Verification items for the finished model (mm, model axes). Round coordinates to 2 decimals unless told otherwise and drop trailing zeros. Write each loop counter-clockwise with the first axis right and the second up, starting at its lowest first coordinate (ties: lowest second). Pieces come first, ordered by that corner, then holes. Notation, with made-up numbers: (46.25, 53) - (51.25, 53) arc R24 cw to (51.25, 69) - close; hole circle Ø6 at (-12, 82.5). An arc over 180 degrees is marked (long way). Answer as a JSON object with one key per item and string values. Group by question number.
1) Go/stop test with flat-tipped pins: pin 1 Ø1.2 at (x, z) = (57, 2.5) entering from +Y; pin 2 Ø1.5 at (x, z) = (29, 0.5) entering from -Y; pin 3 Ø1.5 at (y, z) = (52, 1.5) entering from -X. Record where each tip stops, or that it passes through.
2) Section check C-C (y = 71). Enter the section's corners in (x, z), then the cut area to 3 significant figures.
3) Section check B-B (x = 34.5). Enter the section's corners in (y, z).
4) Thickness scan on line 1 (X direction, y = 21, z = 0.9); line 2 (Y direction, x = 51, z = 3.45); line 3 (X direction, y = 17.5, z = 1.1). Record the ranges inside material, lowest first.
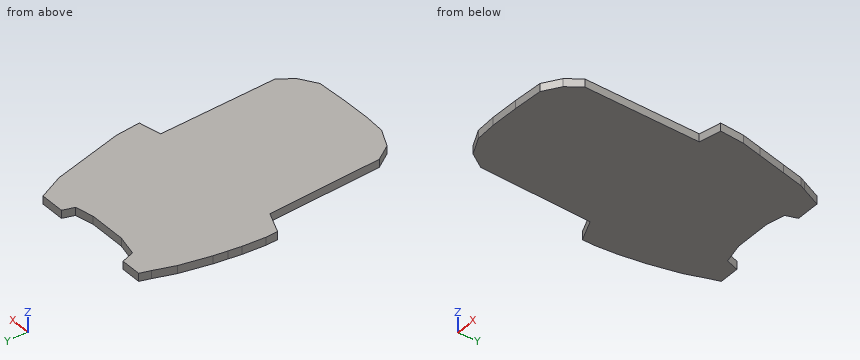
Autodesk Inventor part; units mm, degrees
ref_plane "YZ Plane" through (0, 0, 0) normal (1, 0, 0) x (0, 1, 0)
ref_plane "XZ Plane" through (0, 0, 0) normal (0, 1, 0) x (-1, 0, 0)
ref_plane "XY Plane" through (0, 0, 0) normal (0, 0, 1) x (1, 0, 0)
sketch "Sketch1" plane through (0, 0, 0) normal (0, 0, 1) x (1, 0, 0)
  line L0 (26.9534, 140.31) -> (36.8306, 140.31)
  line L1 (36.8306, 140.31) -> (38.8061, 134.065)
  line L2 (38.8061, 134.065) -> (49.002, 131.6435)
  line L3 (49.002, 131.6435) -> (58.0509, 131.6435)
  line L4 (58.0509, 131.6435) -> (66.8448, 131.6435)
  line L5 (66.8448, 131.6435) -> (75.6388, 133.5552)
  line L6 (75.6388, 133.5552) -> (77.526, 139.065)
  line L7 (77.526, 139.065) -> (89.2513, 139.065)
  line L8 (89.2513, 139.065) -> (93.4636, 129.481)
  line L9 (93.4636, 129.481) -> (94.6369, 126.8115)
  line L10 (94.6369, 126.8115) -> (96.9293, 116.2664)
  line L11 (96.9293, 116.2664) -> (99.976, 102.2517)
  line L12 (99.976, 102.2517) -> (102.1542, 92.2318)
  line L13 (102.1542, 92.2318) -> (102.8007, 80.352)
  line L14 (102.8007, 80.352) -> (92.1232, 78.0307)
  line L15 (92.1232, 78.0307) -> (92.1232, 20.902)
  line L16 (92.1232, 20.902) -> (86.9727, 14.0196)
  line L17 (86.9727, 14.0196) -> (78.9304, 8.8886)
  line L18 (78.9304, 8.8886) -> (64.5453, 8.1057)
  line L19 (64.5453, 8.1057) -> (50.4611, 7.8467)
  line L20 (50.4611, 7.8467) -> (40.2944, 8.4971)
  line L21 (40.2944, 8.4971) -> (31.1734, 13.0172)
  line L22 (31.1734, 13.0172) -> (26.2605, 20.7176)
  line L23 (26.2605, 20.7176) -> (25.2413, 76.1313)
  line L24 (25.2413, 76.1313) -> (14.3454, 80.8506)
  line L25 (14.3454, 80.8506) -> (14.3454, 86.7328)
  line L26 (14.3454, 86.7328) -> (15.5218, 97.7359)
  line L27 (15.5218, 97.7359) -> (16.6126, 103.8324)
  line L28 (16.6126, 103.8324) -> (17.7826, 110.3719)
  line L29 (17.7826, 110.3719) -> (21.4653, 125.2093)
  line L30 (21.4653, 125.2093) -> (25.2413, 135.3116)
  line L31 (25.2413, 135.3116) -> (26.9534, 140.31)
  point P0 (0, 0)
extrude "Extrusion1" add sketch "Sketch1" along normal blind 4
Returned:
{
 "1": {"pin 1": "y = 131.64", "pin 2": "y = 15.25", "pin 3": "x = 25.67"},
 "2": {"outline": "(25.34, 0) - (92.12, 0) - (92.12, 4) - (25.34, 4) - close", "area": "267 mm2"},
 "3": {"outline": "(11.37, 0) - (140.31, 0) - (140.31, 4) - (11.37, 4) - close"},
 "4": {"line 1": "26.26 to 92.12", "line 2": "7.86 to 131.64", "line 3": "28.31 to 89.58"}
}
